Verification items for this drawing (mm, ordinates from the low corner). Coordinates: 2 decimals unless noted, no trailing zeros. Order: outer loops, then holes, each group sorted by start corner. A loop starts at its lowest first (then second) coordinate and runs counter-clockwise, first axis right, second up. Notation, with made-up numbers: (79, 26.5) -> (130, 26.5) arc R34 ccw to (130, 63.5) -> close; hole circle Ø2 at (-5.5, -27). An arc over 180 degrees is marked (long way). Write item = value, one per line. Start each with the question number.
1. Go/stop test with flat-tipped pins: P1, Ø3, axis at y = 34.5, z = 5.5, coming from the -X side; P2, Ø1.5, axis at x = 268, y = 35.5, coming from the +Z side; P3, Ø3, axis at y = 26.5, z = 6, coming from the +X side. Record where each tip stops, or that it passes through.
2. Thickness scan on line 1 along Y through (x, z) = (160, 7.75); line 2 along X through (y, z) = (27.5, 8) (1 decimal); line 3 along X through (y, z) = (27, 5.75) (1 decimal). Record the ranges inside material, lowest first. Write a range as from..to.
3. Cross-section at A-A on x = 160. Record the cut outline in (y, z).
4. Cross-section at B-B on z = 15.5. Record the cut outline in (x, y).
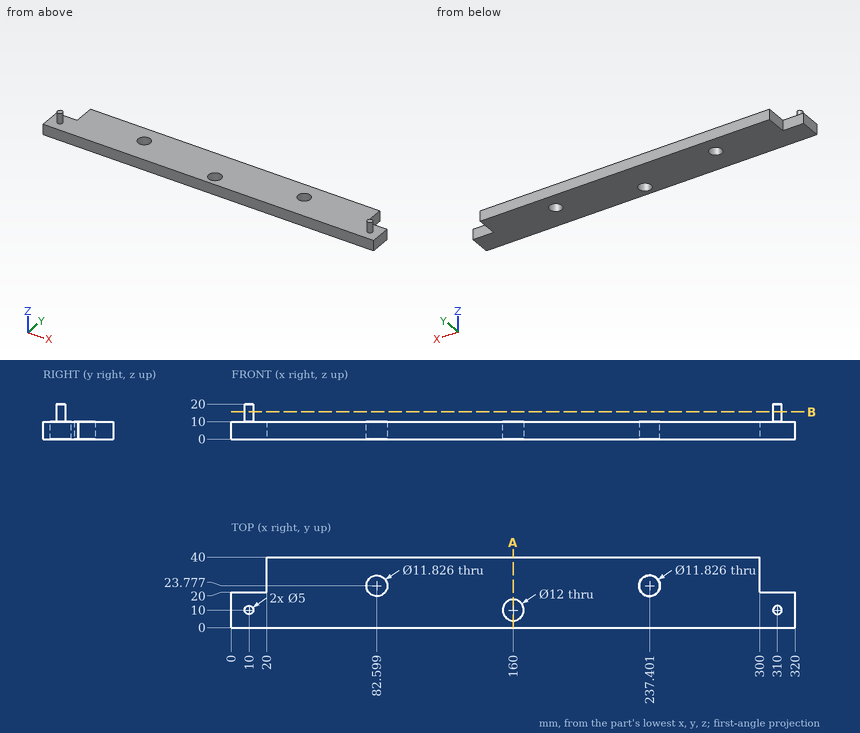
Worked out:
q1.P1 = 20
q1.P2 = 10
q1.P3 = 300
q2.line_1 = 0..4, 16..40
q2.line_2 = 20..78, 87.2..232.8, 242..300
q2.line_3 = 20..77.6, 87.6..232.4, 242.4..300
q3.outline = (0, 0) -> (4, 0) -> (4, 10) -> (0, 10) -> close; (16, 0) -> (40, 0) -> (40, 10) -> (16, 10) -> close
q4.outline = circle Ø5 at (10, 10); circle Ø5 at (310, 10)
